```python
from build123d import *

# Parameters (mm, degrees)
F0_W     = 120
F0_H     = 120
F1_DEPTH = 1400
F2_W     = 40
F2_H     = 175
F3_DEPTH = 120
F4_R     = 5.25
F5_DEPTH = 120.001
F6_R     = 5.25
F7_DEPTH = 120.001


with BuildPart() as f1:
    # F0 (on Top) → F1 (new body, symmetric)
    with BuildSketch(Plane.XY):
        Rectangle(F0_W, F0_H)
    extrude(amount=F1_DEPTH, both=True)

    # F2 (on face) → F3 (cut, through all)
    with BuildSketch(Plane.YZ.offset(60)):
        with Locations((-40, 1312.5)):
            Rectangle(F2_W, F2_H)
    extrude(amount=-F3_DEPTH, mode=Mode.SUBTRACT)

    # F4 (on face) → F5 (cut, through all)
    with BuildSketch(Plane(origin=(0, 60, 0), x_dir=(-1, 0, 0), z_dir=(0, 1, 0))):
        with Locations((0, 1312.5)):
            Circle(F4_R)
        with Locations((0, -1000)):
            Circle(F4_R)
        with Locations((0, 500)):
            Circle(F4_R)
    extrude(amount=-F5_DEPTH, mode=Mode.SUBTRACT)

    # F6 (on face) → F7 (cut, through all)
    with BuildSketch(Plane.YZ.offset(60)):
        with Locations((0, -1050)):
            Circle(F6_R)
        with Locations((0, 600)):
            Circle(F6_R)
    extrude(amount=-F7_DEPTH, mode=Mode.SUBTRACT)


solid = f1.part
```
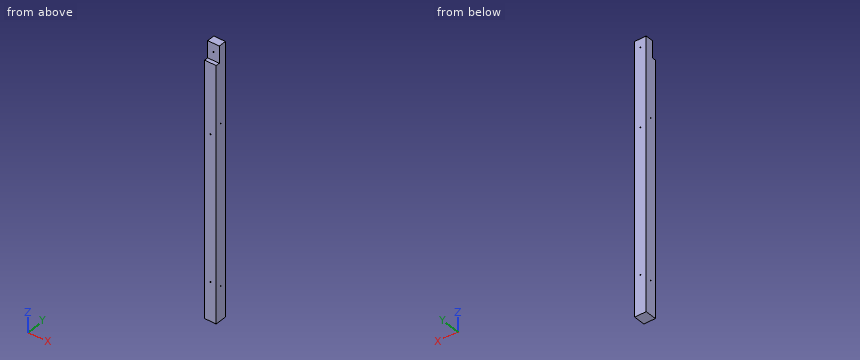
Design review of the part built by this model. Coordinates are the model's own, in mm. Give positions to 0.01 mm unless a question says otherwise; leave off trailing zeros. Write each loop counter-clockwise with the first axis right and the second up, starting at its lowest first coordinate (ties: lowest second). Pieces come first, ordered by that corner, then holes. Notation, with made-up numbers: (48.25, 12) -> (90.25, 12) arc R33 ccw to (90.25, 45) -> close; hole circle Ø7 at (-8.75, -12). An arc over 180 degrees is marked (long way). Answer in a Markdown table with one row per item.
(1) To check wall thickness, follow probe 1 along Z at (x, y) = (0, 8); probe 2 along Z at (x, y) = (-33, 0); probe 3 along X at (y, z) = (-11, 500). State the ranges of each line that lie inside material, in increasing order.
Results:
| item | result |
|---|---|
| probe 1 | -1400 to -1005.25, -994.75 to 494.75, 505.25 to 1307.25, 1317.75 to 1400 |
| probe 2 | -1400 to -1055.25, -1044.75 to 594.75, 605.25 to 1400 |
| probe 3 | -60 to -5.25, 5.25 to 60 |
(2) Consider section A-A (x = 28.5). State the section outline as (y, z) points.
Results:
| item | result |
|---|---|
| outline | (-60, -1400) -> (60, -1400) -> (60, 1400) -> (-20, 1400) -> (-20, 1225) -> (-60, 1225) -> close; hole circle Ø10.5 at (0, -1050); hole circle Ø10.5 at (0, 600) |
(3) Clearance check with flat-ended pins moving along their axes: pin 1 (9.5 mm diameter, centred on x = 0, z = 500, fed in from -Y); pin 2 (12 mm diameter, centred on x = -28, y = -34, fed in from +Z); pin 3 (17 mm diameter, centred on x = 0, z = 1312.5, fed in from -Y). State where each tip first meets the part, or that it passes through.
Results:
| item | result |
|---|---|
| pin 1 | through |
| pin 2 | z = 1225 |
| pin 3 | y = -20 |
